CAD build for the part. Positions are in the model's coordinates, mm. Give positions to 0.01 mm unless a question says otherwise; leave off trailing zeros. Write each loop counter-clockwise with the first axis right and the second up, starting at its lowest first coordinate (ties: lowest second). Pieces come first, ordered by that corner, then holes. Notation, with made-up numbers: (-26.5, -35) -> (-3.5, -35) arc R9 ccw to (-3.5, -31) -> close; hole circle Ø10 at (21, 87.5). An arc over 180 degrees is marked (long way). Answer as a JSON object with one key per item and string values.
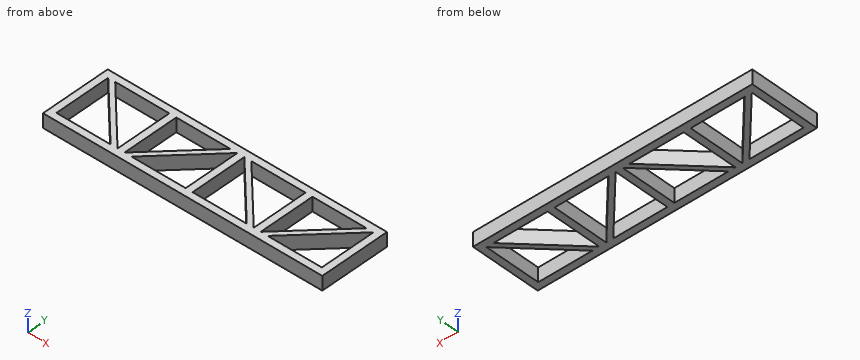
Autodesk Inventor part; units mm, degrees
ref_plane "YZ Plane" through (0, 0, 0) normal (1, 0, 0) x (0, 1, 0)
ref_plane "XZ Plane" through (0, 0, 0) normal (0, 1, 0) x (-1, 0, 0)
ref_plane "XY Plane" through (0, 0, 0) normal (0, 0, 1) x (1, 0, 0)
sketch "Szkic1" plane through (0, 0, 0) normal (0, 0, 1) x (1, 0, 0)
  line L0 (0, 0) -> (200, 0)
  line L1 (0, 0) -> (200, 0)
  line L2 (200, 0) -> (200, 50)
  line L3 (200, 50) -> (0, 50)
  line L4 (0, 50) -> (0, 0)
  line L5 (0, 0) -> (10, 0)
  line L6 (200, 50) -> (195, 50)
  line L7 (200, 50) -> (200, 45)
  line L8 (200, 50) -> (195, 50)
  line L9 (200, 50) -> (200, 45)
  line L10 (195, 45) -> (195, 5)
  line L11 (195, 5) -> (156.25, 5)
  line L12 (5, 5) -> (5, 45)
  line L13 (102.5, 45) -> (102.5, 5)
  line L14 (97.5, 45) -> (97.5, 5)
  line L15 (53.75, 45) -> (53.75, 5)
  line L16 (48.75, 45) -> (48.75, 5)
  line L17 (151.25, 45) -> (151.25, 5)
  line L18 (146.25, 45) -> (146.25, 5)
  line L19 (10, 45) -> (48.75, 5)
  line L20 (43.75, 5) -> (5, 45)
  line L21 (58.75, 5) -> (97.5, 45)
  line L22 (92.5, 45) -> (53.75, 5)
  line L23 (107.5, 45) -> (146.25, 5)
  line L24 (141.25, 5) -> (102.5, 45)
  line L25 (156.25, 5) -> (195, 45)
  line L26 (151.25, 5) -> (190, 45)
  line L27 (10, 45) -> (48.75, 45)
  line L28 (53.75, 45) -> (92.5, 45)
  line L29 (107.5, 45) -> (146.25, 45)
  line L30 (151.25, 45) -> (190, 45)
  line L31 (43.75, 5) -> (5, 5)
  line L32 (97.5, 5) -> (58.75, 5)
  line L33 (141.25, 5) -> (102.5, 5)
  dimension "d2" = 50
extrude "Wyciągnięcie proste1" add sketch "Szkic1" along normal blind 10
properties part number "Kratownica"
1) Wall check: probe 1 along Y at (x, z) = (131.5, 3); probe 2 along Y at (x, z) = (30, 9.5). Give the ranges that are in metal, low to high.
Model answer:
{"probe 1": "y = 0 to 5, 15.06 to 20.23, 45 to 50", "probe 2": "y = 0 to 5, 19.19 to 24.35, 45 to 50"}
2) Slice it at A-A (x = 84.5). List the corners of the cut face in (y, z), then the cut area to 3 significant figures.
Model answer:
{"outline": "(0, 0) -> (5, 0) -> (5, 10) -> (0, 10) -> close; (31.58, 0) -> (36.74, 0) -> (36.74, 10) -> (31.58, 10) -> close; (45, 0) -> (50, 0) -> (50, 10) -> (45, 10) -> close", "area": "152 mm2"}
3) Pin check, flat tip, straight feed: pin 1 (2 mm diameter, centred on x = 62, y = 15, fed in from -Z). Stop position of the tip, or through.
Model answer:
{"pin 1": "passes through"}
4) Slice it at B-B (z = 5.5). State how many separate pieces and enclosed holes the cut face has, then the cut area to 3 significant figures.
Model answer:
{"separate pieces": "1", "enclosed holes": "8", "area": "3,800 mm2"}
5) Slice it at C-C (x = 154). List the corners of the cut face in (y, z).
Model answer:
{"outline": "(0, 0) -> (7.84, 0) -> (7.84, 10) -> (0, 10) -> close; (45, 0) -> (50, 0) -> (50, 10) -> (45, 10) -> close"}
